```python
from build123d import *

# Parameters (mm, degrees)
SKETCH_1_R             = 30
EXTRUDE_1_DEPTH        = 5
SKETCH_2_R             = 5
CUT_EXTRUDE_1_DEPTH    = 93
HOLE_WIZARD_M6_1_D     = 5
HOLE_WIZARD_M6_1_DEPTH = 15
HOLE_WIZARD_M6_1_TIP   = 1.502151548


with BuildPart() as part:
    # 草图1 → 凸台-拉伸1 (new body)
    with BuildSketch(Plane.XY):
        Circle(SKETCH_1_R)
    extrude(amount=EXTRUDE_1_DEPTH)

    # 草图2 → 切除-拉伸1 (cut)
    with BuildSketch(Plane.XY.offset(5)):
        Circle(SKETCH_2_R)
    extrude(amount=-CUT_EXTRUDE_1_DEPTH, mode=Mode.SUBTRACT)

    # M6 螺纹孔1
    with Locations(Plane.XY.offset(5)):
        with Locations((22.5, 0), (0, 22.5), (0, -22.5), (-22.5, 0)):
            Hole(HOLE_WIZARD_M6_1_D / 2, depth=HOLE_WIZARD_M6_1_DEPTH)
            with Locations((0, 0, -(HOLE_WIZARD_M6_1_DEPTH + HOLE_WIZARD_M6_1_TIP / 2))):  # 118° drill point
                Cone(0, HOLE_WIZARD_M6_1_D / 2, HOLE_WIZARD_M6_1_TIP, mode=Mode.SUBTRACT)


solid = part.part
```
The listing builds one solid part. Answer for the finished solid, in the listing's coordinates (mm). Give positions to 0.01 mm unless a question says otherwise; leave off trailing zeros. Write each loop counter-clockwise with the first axis right and the second up, starting at its lowest first coordinate (ties: lowest second). Pieces come first, ordered by that corner, then holes. Notation, with made-up numbers: (-21, 0) -> (10, 0) arc R22 cw to (10, 13) -> close; hole circle Ø2 at (-19.5, 79). An arc over 180 degrees is marked (long way). Use one line per item in the form item = value.
1) Each of these flat-tipped pins is pushed along its axis until it touches: P1, Ø1.5, axis at x = -8, z = 2, coming from the -Y side; P2, Ø1, axis at y = 3.5, z = 3, coming from the +X side; P3, Ø3, axis at y = -23, z = 2.5, coming from the +X side. Where does it stop, or does it pass through?
Result:
P1 = -29.11
P2 = 29.85
P3 = 20.92
2) For a pull along Y with two mould halves and no side action, classify faces 1 (the cylindrical face through (-29.97, 1.32, 2.46)), 2 (the flat face through (6, 0, 5)), 3 (the cylindrical face through (0, -20, 2)) as +Y half, -Y half, draft (parallel to the pull), parting line (faces both ways), or undercut.
Result:
face_1 = parting line
face_2 = draft
face_3 = undercut
3) Section B-B on z = 4.2 is taken. Write down the section's boundary in (x, y).
Result:
outline = circle Ø60 at (0, 0); hole circle Ø5 at (-22.5, 0); hole circle Ø10 at (0, 0); hole circle Ø5 at (0, -22.5); hole circle Ø5 at (0, 22.5); hole circle Ø5 at (22.5, 0)
4) Straight lines are drawn through the part: probe 1 along Y at (x, z) = (0, 3); probe 2 along X at (y, z) = (1.5, 4.4); probe 3 along Y at (x, z) = (-21, 2.15). For each, find the intervals that lie inside material, in ascending order.
Result:
probe_1 = -30 to -25, -20 to -5, 5 to 20, 25 to 30
probe_2 = -29.96 to -24.5, -20.5 to -4.77, 4.77 to 20.5, 24.5 to 29.96
probe_3 = -21.42 to -2, 2 to 21.42
5) Section D-D on x = 22.5 is taken. Write down the section's boundary in (y, z).
Result:
outline = (-19.84, 0) -> (-2.5, 0) -> (-2.5, 5) -> (-19.84, 5) -> close; (2.5, 0) -> (19.84, 0) -> (19.84, 5) -> (2.5, 5) -> close
6) Section A-A on x = 0 is taken. Write down the section's boundary in (y, z), plus the area to 3 significant figures.
Result:
outline = (-30, 0) -> (-25, 0) -> (-25, 5) -> (-30, 5) -> close; (-20, 0) -> (-5, 0) -> (-5, 5) -> (-20, 5) -> close; (5, 0) -> (20, 0) -> (20, 5) -> (5, 5) -> close; (25, 0) -> (30, 0) -> (30, 5) -> (25, 5) -> close
area = 200 mm²
